Input: part model. Units: mm. Frame: model coordinates. Face numbers are marked on the shaded views. A direction names the side the tool comes from. Coordinates: 2 decimals unless noted, no trailing zeros. Order: outer loops, then holes, each group sorted by start corner. A loop starts at its lowest first (then second) coordinate and runs counter-clockwise, first axis right, second up. Notation, with made-up numbers: M 6.5,29 L 62.5,29 A22 cw 62.5,58 Z; hole C 71.5,68.5 d2. An arc over 180 degrees is marked long. One line per item, written item: value.
```python
from build123d import *

# Parameters (mm, degrees)
SALIENTE_EXTRUIR1_DEPTH = 12
SALIENTE_EXTRUIR2_DEPTH = 38
CROQUIS8_W              = 40
CROQUIS8_H              = 20
CORTAR_EXTRUIR5_DEPTH   = 20
CROQUIS3_R              = 4.25
CORTAR_EXTRUIR1_DEPTH   = 13
CORTAR_EXTRUIR2_DEPTH   = 5.5
REDONDEO1_R             = 2
CROQUIS5_W              = 4.8
CROQUIS5_H              = 35
CROQUIS5_W_2            = 15
CROQUIS5_H_2            = 4.8
SALIENTE_EXTRUIR3_DEPTH = 1
NGULO_DE_SALIDA1_ANGLE  = 15
NGULO_DE_SALIDA2_ANGLE  = 15
REDONDEO2_R             = 2
NGULO_DE_SALIDA3_ANGLE  = 15
REDONDEO3_R             = 1
CORTAR_EXTRUIR4_DEPTH   = 66
CORTAR_EXTRUIR6_DEPTH   = 66
CROQUIS12_W             = 65
CROQUIS12_H             = 38
CORTAR_EXTRUIR9_DEPTH   = 66
CROQUIS13_OUTSIDE_W     = 85.54
CROQUIS13_OUTSIDE_H     = 85.54
CROQUIS13_OUTSIDE_W_2   = 55
CROQUIS13_OUTSIDE_H_2   = 35
CORTAR_EXTRUIR10_DEPTH  = 13
REDONDEO5_R             = 2
CROQUIS14_R             = 2.75
CORTAR_EXTRUIR11_DEPTH  = 13


with BuildPart() as part:
    # Croquis1 → Saliente-Extruir1 (new body)
    with BuildSketch(Plane(origin=(0, 0, 0), x_dir=(1, 0, 0), z_dir=(0, 1, 0))):
        Polygon((25, 65), (25, 25), (65, 25), (65, 0), (0, 0), (0, 65), align=None)
    extrude(amount=SALIENTE_EXTRUIR1_DEPTH)

    # Croquis2 → Saliente-Extruir2 (add)
    with BuildSketch(Plane(origin=(0, 12, 0), x_dir=(1, 0, 0), z_dir=(0, 1, 0))):
        Polygon((0, 65), (0, 0), (65, 0), (65, 5), (37.4, 5), (37.4, 6), (32.6, 6), (32.6, 5), (17.4, 5), (17.4, 6), (12.6, 6), (12.6, 5), (5, 5), (5, 12.6), (6, 12.6), (6, 17.4), (5, 17.4), (5, 65), align=None)
    extrude(amount=SALIENTE_EXTRUIR2_DEPTH)

    # Croquis8 → Cortar-Extruir5 (cut)
    with BuildSketch(Plane(origin=(0, 50, 0), x_dir=(1, 0, 0), z_dir=(0, 1, 0))):
        with Locations((25, 15)):
            Rectangle(CROQUIS8_W, CROQUIS8_H)
    extrude(amount=-CORTAR_EXTRUIR5_DEPTH, mode=Mode.SUBTRACT)

    # Croquis3 → Cortar-Extruir1 (cut, through all)
    with BuildSketch(Plane(origin=(0, 12, 0), x_dir=(1, 0, 0), z_dir=(0, 1, 0))):
        with Locations((25, 15)):
            Circle(CROQUIS3_R)
    extrude(amount=-CORTAR_EXTRUIR1_DEPTH, mode=Mode.SUBTRACT)

    # Croquis4 → Cortar-Extruir2 (cut)
    with BuildSketch(Plane(origin=(0, 12, 0), x_dir=(1, 0, 0), z_dir=(0, 1, 0))):
        Polygon((32.621023553, 15), (28.810511777, 21.6), (21.189488223, 21.6), (17.378976447, 15), (21.189488223, 8.4), (28.810511777, 8.4), align=None)
    extrude(amount=-CORTAR_EXTRUIR2_DEPTH, mode=Mode.SUBTRACT)

    # Redondeo1
    redondeo1_edges = [part.edges().sort_by_distance(p)[0] for p in [
        (25, 6, -25),
    ]]
    fillet(redondeo1_edges, radius=REDONDEO1_R)

    # Croquis5 → Saliente-Extruir3 (add)
    with BuildSketch(Plane(origin=(0, 12, 0), x_dir=(1, 0, 0), z_dir=(0, 1, 0))):
        with Locations((15, 47.5)):
            Rectangle(CROQUIS5_W, CROQUIS5_H)
        with Locations((57.5, 15)):
            Rectangle(CROQUIS5_W_2, CROQUIS5_H_2)
    extrude(amount=SALIENTE_EXTRUIR3_DEPTH)

    # Ángulo de salida1
    ngulo_de_salida1_faces = [part.faces().sort_by_distance(p)[0] for p in [
        (57.5, 12.5, -17.4),
        (50, 12.5, -15),
        (57.5, 12.5, -12.6),
        (12.6, 12.5, -47.5),
        (15, 12.5, -30),
        (17.4, 12.5, -47.5),
    ]]
    draft(ngulo_de_salida1_faces, Plane.ZX.offset(12), NGULO_DE_SALIDA1_ANGLE)

    # Ángulo de salida2
    ngulo_de_salida2_faces = [part.faces().sort_by_distance(p)[0] for p in [
        (15, 30, -5.5),
        (35, 30, -5.5),
        (37.4, 21, -5.5),
        (32.6, 21, -5.5),
        (17.4, 21, -5.5),
        (12.6, 21, -5.5),
    ]]
    draft(ngulo_de_salida2_faces, Plane(origin=(65, 50, -5), x_dir=(-1, 0, 0), z_dir=(0, 0, -1)), NGULO_DE_SALIDA2_ANGLE)

    # Redondeo2
    redondeo2_edges = [part.edges().sort_by_distance(p)[0] for p in [
        (0, 25, 0),
    ]]
    fillet(redondeo2_edges, radius=REDONDEO2_R)

    # Ángulo de salida3
    ngulo_de_salida3_faces = [part.faces().sort_by_distance(p)[0] for p in [
        (5.5, 30, -15),
        (5.5, 21, -17.4),
        (5.5, 21, -12.6),
    ]]
    draft(ngulo_de_salida3_faces, Plane(origin=(5, 50, -5), x_dir=(0, 0, 1), z_dir=(1, 0, 0)), NGULO_DE_SALIDA3_ANGLE)

    # Redondeo3
    redondeo3_edges = [part.edges().sort_by_distance(p)[0] for p in [
        (5, 31, -5),
    ]]
    fillet(redondeo3_edges, radius=REDONDEO3_R)

    # Croquis6 → Cortar-Extruir4 (cut, through all)
    with BuildSketch(Plane.ZY):
        with BuildLine():
            Line((-16, 45.5), (-14, 45.5))
            Line((-14, 45.5), (-12.696855696, 43.502673056))
            ThreePointArc((-12.696855696, 43.502673056), (-15, 39.25), (-17.303144304, 43.502673056))
            Line((-17.303144304, 43.502673056), (-16, 45.5))
        make_face()
        with BuildLine():
            Line((-56, 45.5), (-54, 45.5))
            Line((-54, 45.5), (-52.696855696, 43.502673056))
            ThreePointArc((-52.696855696, 43.502673056), (-55, 39.25), (-57.303144304, 43.502673056))
            Line((-57.303144304, 43.502673056), (-56, 45.5))
        make_face()
        with BuildLine():
            Line((-56, 25.5), (-54, 25.5))
            Line((-54, 25.5), (-52.696855696, 23.502673056))
            ThreePointArc((-52.696855696, 23.502673056), (-55, 19.25), (-57.303144304, 23.502673056))
            Line((-57.303144304, 23.502673056), (-56, 25.5))
        make_face()
    extrude(amount=-CORTAR_EXTRUIR4_DEPTH, mode=Mode.SUBTRACT)

    # Croquis9 → Cortar-Extruir6 (cut, through all)
    with BuildSketch(Plane.XY):
        with BuildLine():
            Line((14, 45.5), (16, 45.5))
            Line((16, 45.5), (17.303144304, 43.502673056))
            ThreePointArc((17.303144304, 43.502673056), (15, 39.25), (12.696855696, 43.502673056))
            Line((12.696855696, 43.502673056), (14, 45.5))
        make_face()
        with BuildLine():
            Line((54, 45.5), (56, 45.5))
            Line((56, 45.5), (57.303144304, 43.502673056))
            ThreePointArc((57.303144304, 43.502673056), (55, 39.25), (52.696855696, 43.502673056))
            Line((52.696855696, 43.502673056), (54, 45.5))
        make_face()
        with BuildLine():
            Line((54, 25.5), (56, 25.5))
            Line((56, 25.5), (57.303144304, 23.502673056))
            ThreePointArc((57.303144304, 23.502673056), (55, 19.25), (52.696855696, 23.502673056))
            Line((52.696855696, 23.502673056), (54, 25.5))
        make_face()
    extrude(amount=-CORTAR_EXTRUIR6_DEPTH, mode=Mode.SUBTRACT)

    # Croquis12 → Cortar-Extruir9 (cut, through all)
    with BuildSketch(Plane(origin=(65, 0, 0), x_dir=(0, 0, -1), z_dir=(1, 0, 0))):
        with Locations((32.5, 31)):
            Rectangle(CROQUIS12_W, CROQUIS12_H)
    extrude(amount=-CORTAR_EXTRUIR9_DEPTH, mode=Mode.SUBTRACT)

    # Croquis13 outside → Cortar-Extruir10 (cut, through all)
    with BuildSketch(Plane(origin=(0, 12, 0), x_dir=(1, 0, 0), z_dir=(0, 1, 0))):
        with Locations((32.5, 32.5)):
            Rectangle(CROQUIS13_OUTSIDE_W, CROQUIS13_OUTSIDE_H)
        with Locations((32.5, 22.5)):
            Rectangle(CROQUIS13_OUTSIDE_W_2, CROQUIS13_OUTSIDE_H_2, mode=Mode.SUBTRACT)
    extrude(amount=-CORTAR_EXTRUIR10_DEPTH, mode=Mode.SUBTRACT)

    # Redondeo5
    redondeo5_edges = [part.edges().sort_by_distance(p)[0] for p in [
        (5, 6, -5),
    ]]
    fillet(redondeo5_edges, radius=REDONDEO5_R)

    # Croquis14 → Cortar-Extruir11 (cut, through all)
    with BuildSketch(Plane(origin=(0, 12, 0), x_dir=(1, 0, 0), z_dir=(0, 1, 0))):
        with Locations((15, 30)):
            Circle(CROQUIS14_R)
        with Locations((50, 15)):
            Circle(CROQUIS14_R)
    extrude(amount=-CORTAR_EXTRUIR11_DEPTH, mode=Mode.SUBTRACT)


solid = part.part
```
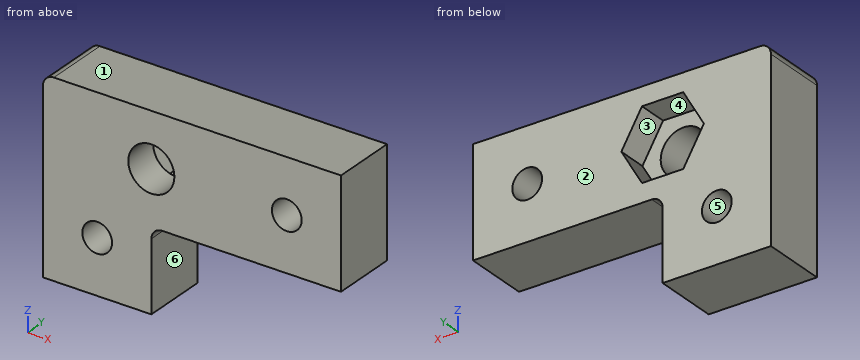
(1) Cut plane C-C on y = 10.5. Output: boundary loops of the cut face in (x, z), plus the area to 3 significant figures.
Data:
outline: M 5,-40 L 25,-40 L 25,-27 A2 cw 27,-25 L 60,-25 L 60,-5 L 7,-5 A2 ccw 5,-7 Z; hole C 15,-30 d5.5; hole M 17.38,-15 L 21.19,-21.6 L 28.81,-21.6 L 32.62,-15 L 28.81,-8.4 L 21.19,-8.4 Z; hole C 50,-15 d5.5
area: 1,200 mm2
(2) Cut plane A-A on x = 15. Output: boundary loops of the cut face in (y, z).
Data:
outline: M 0,-40 L 12,-40 L 12,-32.75 L 0,-32.75 Z; M 0,-27.25 L 12,-27.25 L 12,-5 L 0,-5 Z
(3) First-contact query: pin 1 (1 mm diameter, centred on x = 28.5, y = 7.5, fed in from -Z); pin 2 (6.5 mm diameter, centred on x = 50, z = -15, fed in from +Y). Flat tips, straight axial feed; report the tip coordinate or a pass-through.
Data:
pin 1: stops at z = -25
pin 2: stops at y = 12
(4) Cut plane D-D on z = -16.5. Output: boundary loops of the cut face in (x, y) (1 decimal), plus the area to 3 significant figures.
Data:
outline: M 5,0 L 21,0 L 21,6.5 L 18.2,6.5 L 18.2,12 L 5,12 Z; M 29,0 L 47.7,0 L 47.7,12 L 31.8,12 L 31.8,6.5 L 29,6.5 Z; M 52.3,0 L 60,0 L 60,12 L 52.3,12 Z
area: 479 mm2
(5) Draft query along Z for the marked faces 1, 2 and 3. Return one class per face: released by +Z, released by -Z, zero draft, split by the parting line, or undercut.
Data:
face 1: released by +Z
face 2: zero draft
face 3: undercut
(6) Ray query, line 1 (X direction, y = 4.75, z = -15); line 2 (X direction, y = 7.75, z = -15); line 3 (X direction, y = 4.5, z = -30). Return the intervals inside material, ascending. Write a range as from..to.
Data:
line 1: x = 5..20.75, 29.25..47.25, 52.75..60
line 2: x = 5..17.38, 32.62..47.25, 52.75..60
line 3: x = 5..12.25, 17.75..25
(7) Cut plane B-B on z = -30. Output: boundary loops of the cut face in (x, y).
Data:
outline: M 5,0 L 12.25,0 L 12.25,12 L 5,12 Z; M 17.75,0 L 25,0 L 25,12 L 17.75,12 Z
(8) Access query for the marked faces 4, 5 and 6. Directions: +Z, -Z, +X, -X, +Y, -Y. A direction counts if a zero-diameter tool reaches every point of the face in a straight line with its end or side. Return the directions, or none.
Data:
face 4: +Y
face 5: +Y, -Y
face 6: -Z, +X, +Y, -Y
